Check sheet for the modelled part. Datum: model origin and axes. Units: mm. A direction names the side the tool comes from. Coordinates: 2 decimals unless noted, no trailing zeros. Loops run counter-clockwise (first coordinate to the right, second up) from the corner with the lowest first, then second, coordinate; pieces in that order, holes last. Notation, with made-up numbers: M 71,-9 L 101,-9 A11 ccw 101,-3 Z; hole C -22.75,82.5 d8. An arc over 180 degrees is marked long. Return JSON: item names as keys, results as strings.
from build123d import *

# Parameters (mm, degrees)
F1_DEPTH = 5
F2_W     = 20
F2_H     = 10
F3_DEPTH = 10


with BuildPart() as f1:
    # F0 (on Front) → F1 (new body)
    with BuildSketch(Plane.XZ):
        Polygon((0, 35), (0, 0), (10, 0), (20, 0), (20, 35), (14, 35), (10, 10), (6, 35), align=None)
    extrude(amount=F1_DEPTH)

    # F2 (on face) → F3 (join)
    with BuildSketch(Plane.XZ.offset(5)):
        with Locations((10, 5)):
            Rectangle(F2_W, F2_H)
    extrude(amount=F3_DEPTH)

    # F4: F1 across face


with BuildPart() as f1_1:
    add(f1.part)
    add(f1.part.mirror(Plane(origin=(10, -15, 5), x_dir=(1, 0, 0), z_dir=(0, -1, 0))))


solid = f1_1.part
1) Section check B-B on x = 12. Record the cut outline in (y, z).
Answers:
{"outline": "M -30,0 L 0,0 L 0,22.5 L -5,22.5 L -5,10 L -25,10 L -25,22.5 L -30,22.5 Z"}
2) Section check C-C on y = -25.5. Record the cut outline in (x, z), then the cut area to 3 significant figures.
Answers:
{"outline": "M 0,0 L 20,0 L 20,35 L 14,35 L 10,10 L 6,35 L 0,35 Z", "area": "600 mm²"}
3) Go/stop test with a flat-tipped pin: pin 1 Ø5 at (x, y) = (17.5, -17) entering from +Z. Record where the tip stops, or that it passes through.
Answers:
{"pin 1": "z = 10"}
4) Section check D-D on z = 11. Record the cut outline in (x, y), then the cut area to 3 significant figures.
Answers:
{"outline": "M 0,-30 L 9.84,-30 L 9.84,-25 L 0,-25 Z; M 0,-5 L 9.84,-5 L 9.84,0 L 0,0 Z; M 10.16,-30 L 20,-30 L 20,-25 L 10.16,-25 Z; M 10.16,-5 L 20,-5 L 20,0 L 10.16,0 Z", "area": "197 mm²"}
5) Draft check along Y on faces 1 (the face through (12, -30, 18)), 2 (the face through (10, -15, 10)), 3 (the face through (3, -28, 35)). Enter one of: +Y half, -Y half, draft (parallel to the pull), parting line (faces both ways), or undercut.
Answers:
{"face 1": "-Y half", "face 2": "undercut", "face 3": "draft"}
6) Set-up check for faces 4 (the face through (12.028, -27.535, 22.675)), 5 (the face through (0, -15, 9)), 6 (the face through (4, -25, 23)): record each of +Z, -Z, +X, -X, +Y, -Y from which the full face is reachable in a straight line by a thin tool's end or side.
Answers:
{"face 4": "+Z, +Y, -Y", "face 5": "+Z, -Z, -X, +Y, -Y", "face 6": "+Z, +X, -X"}
7) Section check A-A on z = 21. Record the cut outline in (x, y).
Answers:
{"outline": "M 0,-30 L 8.24,-30 L 8.24,-25 L 0,-25 Z; M 0,-5 L 8.24,-5 L 8.24,0 L 0,0 Z; M 11.76,-30 L 20,-30 L 20,-25 L 11.76,-25 Z; M 11.76,-5 L 20,-5 L 20,0 L 11.76,0 Z"}
8) Scan lines: line 1 along Y through (x, z) = (5.75, 15); line 2 along Z through (x, y) = (9, -21); line 3 along X through (y, z) = (-1.5, 25). Record each from-to range of solid material in increasing order. Write a range as [from, to].
Answers:
{"line 1": "[-30, -25], [-5, 0]", "line 2": "[0, 10]", "line 3": "[0, 7.6], [12.4, 20]"}
